Build history of the part. All positions in model axes, mm. Round coordinates to 2 decimals unless told otherwise and drop trailing zeros. Loops run counter-clockwise (first coordinate to the right, second up) from the corner with the lowest first, then second, coordinate; pieces in that order, holes last. Notation, with made-up numbers: (79.5, 45.25) - (104.5, 45.25) arc R17 cw to (104.5, 70.25) - close; hole circle Ø6 at (9.5, 72). An arc over 180 degrees is marked (long way). One line per question, with ' | ' between items. Start each with the question number.
from build123d import *

# Parameters (mm, degrees)
SKETCH1_W             = 110
SKETCH1_H             = 46
BOSS_EXTRUDE1_DEPTH   = 6.35
SKETCH5_R             = 5
CUT_EXTRUDE1_DEPTH    = 7.35
SKETCH7_R             = 4
CUT_EXTRUDE2_DEPTH    = 7.35
FILLET1_R             = 5
F_8_32_TAPPED_HOLE1_D = 3.4544
F_8_CLEARANCE_HOLE1_D = 4.3053
F_6_CLEARANCE_HOLE2_D = 3.6576


with BuildPart() as part:
    # Sketch1 → Boss-Extrude1 (new body)
    with BuildSketch(Plane.XY):
        Rectangle(SKETCH1_W, SKETCH1_H)
    extrude(amount=BOSS_EXTRUDE1_DEPTH)

    # Sketch5 → Cut-Extrude1 (cut, through all)
    with BuildSketch(Plane(origin=(0, 0, 0), x_dir=(-1, 0, 0), z_dir=(0, 0, -1))):
        with Locations((-10, -5)):
            Circle(SKETCH5_R)
        with Locations((10, -5)):
            Circle(SKETCH5_R)
    extrude(amount=-CUT_EXTRUDE1_DEPTH, mode=Mode.SUBTRACT)

    # Sketch7 → Cut-Extrude2 (cut, through all)
    with BuildSketch(Plane(origin=(0, 0, 0), x_dir=(-1, 0, 0), z_dir=(0, 0, -1))):
        with Locations((-23, 8)):
            Circle(SKETCH7_R)
        with Locations((-23, -8)):
            Circle(SKETCH7_R)
        with Locations((23, -8)):
            Circle(SKETCH7_R)
        with Locations((23, 8)):
            Circle(SKETCH7_R)
        with Locations((-47, 8)):
            Circle(SKETCH7_R)
        with Locations((-47, -8)):
            Circle(SKETCH7_R)
        with Locations((47, 8)):
            Circle(SKETCH7_R)
        with Locations((47, -8)):
            Circle(SKETCH7_R)
    extrude(amount=-CUT_EXTRUDE2_DEPTH, mode=Mode.SUBTRACT)

    # Fillet1
    fillet1_edges = [part.edges().sort_by_distance(p)[0] for p in [
        (-55, -23, 3.175),
        (-55, 23, 3.175),
        (55, 23, 3.175),
        (55, -23, 3.175),
    ]]
    fillet(fillet1_edges, radius=FILLET1_R)

    # #8-32 Tapped Hole1 (through all)
    with Locations(Plane(origin=(0, 0, 0), x_dir=(-1, 0, 0), z_dir=(0, 0, -1))):
        with Locations((-23, 19), (23, 19), (23, -19), (-23, -19)):
            Hole(F_8_32_TAPPED_HOLE1_D / 2)

    # #8 Clearance Hole1 (through all)
    with Locations(Plane(origin=(0, 0, 0), x_dir=(-1, 0, 0), z_dir=(0, 0, -1))):
        with Locations((-50, 19), (-50, -19), (50, -19), (50, 19)):
            Hole(F_8_CLEARANCE_HOLE1_D / 2)

    # #6 Clearance Hole2 (through all)
    with Locations(Plane(origin=(0, 0, 0), x_dir=(-1, 0, 0), z_dir=(0, 0, -1))):
        with Locations((-35, 10), (-35, -10), (35, -10), (35, 10)):
            Hole(F_6_CLEARANCE_HOLE2_D / 2)


solid = part.part
1) Wall check: line 1 (Y direction, x = -23, z = 2.75); line 2 (Y direction, x = 34.5, z = 2.5); line 3 (X direction, y = 5.5, z = 4.25). Give the ranges that are in metal, low to high. Write a range as [from, to].
2) Saw through at C-C on z = 5.25. State how many separate pieces and enclosed holes the cut face has, and give its area (3 significant figures).
3) Drop a flat-ended pin along its axis: pin 1 (5 mm diameter, centred on x = -35, y = 10, fed in from -Z). Give the stop position or say it passes through.
4) Two-plate mould, pull along X, no slides. Class faces 1 (the flat face through (55, 0, 3)), 2 (the cylindrical face through (-23.225, -17.287, 3.219)), 3 (the cylindrical face through (36.744, 10.549, 3.219)), 4 (the flat face through (-1, 23, 3)): +X half, -X half, draft (parallel to the pull), parting line (faces both ways), or undercut.
5) Saw through at A-A on x = 13. Write the cut outline in (y, z), and give its area (3 significant figures).
6) Saw through at B-B on x = -35. Write the cut outline in (y, z).
Answer key:
1) line 1: [-23, -20.73], [-17.27, -12], [-4, 4], [12, 17.27], [20.73, 23] | line 2: [-23, -11.76], [-8.24, 8.24], [11.76, 23] | line 3: [-55, -50.12], [-43.88, -26.12], [-19.88, 19.88], [26.12, 43.88], [50.12, 55]
2) separate pieces: 1 | enclosed holes: 22 | area: 4,340 mm²
3) pin 1: z = 0
4) face 1: +X half | face 2: undercut | face 3: undercut | face 4: draft
5) outline: (-23, 0) - (-9, 0) - (-9, 6.35) - (-23, 6.35) - close; (-1, 0) - (23, 0) - (23, 6.35) - (-1, 6.35) - close | area: 241 mm²
6) outline: (-23, 0) - (-11.83, 0) - (-11.83, 6.35) - (-23, 6.35) - close; (-8.17, 0) - (8.17, 0) - (8.17, 6.35) - (-8.17, 6.35) - close; (11.83, 0) - (23, 0) - (23, 6.35) - (11.83, 6.35) - close
